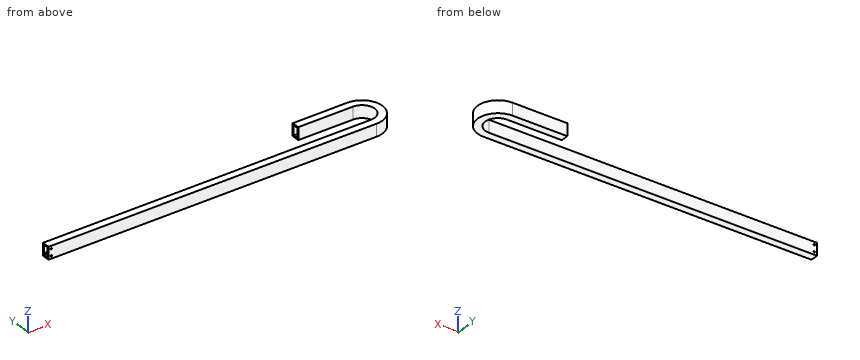
```python
from build123d import *

# Parameters (mm, degrees)
SKETCH_2_W              = 45
SKETCH_2_H              = 28
SKETCH_2_W_2            = 35
SKETCH_2_H_2            = 18
HOLE_WIZARD_5_5_5_5_1_D = 5.5


with BuildPart() as part:
    # 扫描1: sweep along a path in 草图1
    with BuildLine(Plane.XY) as sweep_1_path:
        Line((0, 0), (1200, 0))
        ThreePointArc((1200, 0), (1260, 60), (1200, 120))
        Line((1200, 120), (1000, 120))
    # 草图2 → 扫描1 (sweep)
    with BuildSketch(Plane(origin=(0, 0, 0), x_dir=(0, 0, -1), z_dir=(1, 0, 0))):
        Rectangle(SKETCH_2_W, SKETCH_2_H)
        Rectangle(SKETCH_2_W_2, SKETCH_2_H_2, mode=Mode.SUBTRACT)
    sweep(path=sweep_1_path.line)

    # Ø5.5 (5.5) 直径孔1 (through all)
    with Locations(Plane(origin=(10, 14, -12.5), x_dir=(0, 0, 1), z_dir=(0, 1, 0))):
        with Locations((0, 0), (25, 0)):
            Hole(HOLE_WIZARD_5_5_5_5_1_D / 2)


solid = part.part
```
Could you check a few things on this model? Use its own coordinates, in mm. Give positions to 0.01 mm unless a question says otherwise; leave off trailing zeros. Order: outer loops, then holes, each group sorted by start corner. A loop starts at its lowest first (then second) coordinate and runs counter-clockwise, first axis right, second up.
Q1. Suppose I cut it at A-A, the plane x = 807. Write out the boundary of the cut face in (y, z), and give its area (3 significant figures).
Q2. Suppose I cut it at B-B, the plane z = -2.5. Write out the boundary of the cut face in (x, y), and give its area (3 significant figures).
Q3. Suppose I cut it at C-C, the plane y = 60. Write out the boundary of the cut face in (x, z), and give its area (3 significant figures).
Q4. If I drill on line 1 along Y through (x, z) = (1158.5, 14.5); line 2 along Z through (x, y) = (404, 5); line 3 along Y through (x, z) = (992.5, 9), over which ranges is the centre line in solid material (lowest first)?
Q5. I'm going to push flat-ended pins straight in: P1, Ø3, axis at y = 67.5, z = -11, coming from the -X side; P2, Ø2, axis at y = 19.5, z = 9.5, coming from the +X side; P3, Ø8, axis at y = 75.5, z = -14.5, coming from the +X side. Where does each tip first touch, or does it pass through?
Solution:
1. outline: (-14, -22.5) - (14, -22.5) - (14, 22.5) - (-14, 22.5) - close; hole (-9, -17.5) - (9, -17.5) - (9, 17.5) - (-9, 17.5) - close
1. area: 630 mm2
2. outline: (0, -14) - (1200, -14) arc R74 ccw to (1200, 134) - (1000, 134) - (1000, 129) - (1200, 129) arc R69 cw to (1200, -9) - (0, -9) - close; (0, 9) - (1200, 9) arc R51 ccw to (1200, 111) - (1000, 111) - (1000, 106) - (1200, 106) arc R46 cw to (1200, 14) - (0, 14) - close
2. area: 15,900 mm2
3. outline: (1246, -22.5) - (1274, -22.5) - (1274, 22.5) - (1246, 22.5) - close; hole (1251, -17.5) - (1269, -17.5) - (1269, 17.5) - (1251, 17.5) - close
3. area: 630 mm2
4. line 1: y = -14 to -9, 9 to 14, 106 to 111, 129 to 134
4. line 2: z = -22.5 to -17.5, 17.5 to 22.5
4. line 3: y = -14 to -9, 9 to 14
5. P1: stops at x = 1245.11
5. P2: stops at x = 1262.58
5. P3: stops at x = 1273.1
